The listing builds one solid part. Answer for the finished solid, in the listing's coordinates (mm). A direction names the side the tool comes from. Round coordinates to 2 decimals unless told otherwise and drop trailing zeros. Write each loop counter-clockwise with the first axis right and the second up, starting at its lowest first coordinate (ties: lowest second). Pieces come first, ordered by that corner, then holes. Notation, with made-up numbers: (64, -38) - (85, -38) arc R37 cw to (85, 1) - close; hole circle Ø5 at (19, -12.75). An arc over 180 degrees is marked (long way). Answer in a Markdown table with one row per item.
from build123d import *

# Parameters (mm, degrees)
SKETCH1_W           = 40
SKETCH1_H           = 35
SKETCH1_R           = 2.25
SKETCH1_W_2         = 6
SKETCH1_H_2         = 25
BOSS_EXTRUDE1_DEPTH = 4
SKETCH2_W           = 6
SKETCH2_H           = 25
BOSS_EXTRUDE2_DEPTH = 26
SKETCH3_R           = 2.35
CUT_EXTRUDE1_DEPTH  = 45.760529843
FILLET1_R           = 10
CHAMFER1_SIZE       = 1


with BuildPart() as part:
    # Sketch1 → Boss-Extrude1 (new body)
    with BuildSketch(Plane(origin=(0, 0, 0), x_dir=(1, 0, 0), z_dir=(0, 1, 0))):
        with Locations((-0.498134051, -0.87173459)):
            Rectangle(SKETCH1_W, SKETCH1_H)
        with Locations(Location((-12.118134051, -9.62173459, 0), (0, 0, 270))):
            Circle(SKETCH1_R, mode=Mode.SUBTRACT)
        with Locations(Location((-12.118134051, 7.87826541, 0), (0, 0, 270))):
            Circle(SKETCH1_R, mode=Mode.SUBTRACT)
        with Locations((10.881865949, -0.87173459)):
            Rectangle(SKETCH1_W_2, SKETCH1_H_2, mode=Mode.SUBTRACT)
    extrude(amount=BOSS_EXTRUDE1_DEPTH)

    # Sketch2 → Boss-Extrude2 (add)
    with BuildSketch(Plane(origin=(0, 4, 0), x_dir=(1, 0, 0), z_dir=(0, 1, 0))):
        with Locations((10.881865949, -0.87173459)):
            Rectangle(SKETCH2_W, SKETCH2_H)
    extrude(amount=-BOSS_EXTRUDE2_DEPTH)

    # Sketch3 → Cut-Extrude1 (cut, through all)
    with BuildSketch(Plane(origin=(13.881865949, 0, 0), x_dir=(0, 0, -1), z_dir=(1, 0, 0))):
        with Locations((6.12826541, -16.5)):
            Circle(SKETCH3_R)
        with Locations(Location((-7.87173459, -16.5, 0), (0, 0, 180))):
            Circle(SKETCH3_R)
    extrude(amount=-CUT_EXTRUDE1_DEPTH, mode=Mode.SUBTRACT)

    # Fillet1
    fillet1_edges = [part.edges().sort_by_distance(p)[0] for p in [
        (19.501865949, 2, 18.37173459),
        (-20.498134051, 2, 18.37173459),
        (-20.498134051, 2, -16.62826541),
        (19.501865949, 2, -16.62826541),
    ]]
    fillet(fillet1_edges, radius=FILLET1_R)

    # Chamfer1
    chamfer1_edges = [part.edges().sort_by_distance(p)[0] for p in [
        (-12.118134051, 0, 7.37173459),
        (-12.118134051, 4, 7.37173459),
        (-12.118134051, 0, -10.12826541),
        (-12.118134051, 4, -10.12826541),
        (7.881865949, -11, -11.62826541),
        (10.881865949, -22, -11.62826541),
        (13.881865949, -11, -11.62826541),
        (13.881865949, -22, 0.87173459),
        (13.881865949, -11, 13.37173459),
        (10.881865949, -22, 13.37173459),
        (7.881865949, -11, 13.37173459),
        (7.881865949, -22, 0.87173459),
        (7.881865949, -16.5, -3.77826541),
        (13.881865949, -16.5, -3.77826541),
        (7.881865949, -16.5, 5.52173459),
        (13.881865949, -16.5, 5.52173459),
        (19.501865949, 0, 0.87173459),
        (19.501865949, 4, 0.87173459),
        (-0.498134051, 0, 18.37173459),
        (-20.498134051, 0, 0.87173459),
        (-0.498134051, 0, -16.62826541),
        (-17.569201863, 0, 15.442802401),
        (-17.569201863, 0, -13.699333222),
        (16.572933761, 0, -13.699333222),
        (16.572933761, 0, 15.442802401),
        (-0.498134051, 4, 18.37173459),
        (-0.498134051, 4, -16.62826541),
        (-20.498134051, 4, 0.87173459),
        (-17.569201863, 4, 15.442802401),
        (-17.569201863, 4, -13.699333222),
        (16.572933761, 4, -13.699333222),
        (16.572933761, 4, 15.442802401),
    ]]
    chamfer(chamfer1_edges, length=CHAMFER1_SIZE)


solid = part.part
(1) Section B-B (z = -2) is taken. Give the vertices of the cut face in (x, y).
Checked values:
| item | result |
|---|---|
| outline | (-20.5, 1) - (-19.5, 0) - (7.88, 0) - (7.88, -21) - (8.88, -22) - (12.88, -22) - (13.88, -21) - (13.88, 0) - (18.5, 0) - (19.5, 1) - (19.5, 3) - (18.5, 4) - (-19.5, 4) - (-20.5, 3) - close |
(2) Section A-A (y = -16.5) is taken. Give the vertices of the cut face in (x, z).
Checked values:
| item | result |
|---|---|
| outline | (7.88, -10.63) - (8.88, -11.63) - (12.88, -11.63) - (13.88, -10.63) - (13.88, -9.48) - (12.88, -8.48) - (8.88, -8.48) - (7.88, -9.48) - close; (7.88, -2.78) - (8.88, -3.78) - (12.88, -3.78) - (13.88, -2.78) - (13.88, 4.52) - (12.88, 5.52) - (8.88, 5.52) - (7.88, 4.52) - close; (7.88, 11.22) - (8.88, 10.22) - (12.88, 10.22) - (13.88, 11.22) - (13.88, 12.37) - (12.88, 13.37) - (8.88, 13.37) - (7.88, 12.37) - close |
(3) For faces 4 (the flat face through (13.882, -10, 1)), 5 (the flat face through (13.389, -10.353, 12.865)), 6 (the flat face through (-0.36, 0.51, -16.14)), determine the directions among +Z, -Z, +X, -X, +Y, -Y from which every point of the face is accessible in a straight line to the end or side of a thin tool.
Checked values:
| item | result |
|---|---|
| face 4 | +Z, -Z, +X, -Y |
| face 5 | +Z, +X, -Y |
| face 6 | -Z, +X, -X, -Y |
(4) Section C-C (y = -3) is taken. Give the vertices of the cut face in (x, z).
Checked values:
| item | result |
|---|---|
| outline | (7.88, -10.63) - (8.88, -11.63) - (12.88, -11.63) - (13.88, -10.63) - (13.88, 12.37) - (12.88, 13.37) - (8.88, 13.37) - (7.88, 12.37) - close |
(5) Section D-D (x = -7) is taken. Give the vertices of the cut face in (y, z).
Checked values:
| item | result |
|---|---|
| outline | (0, -15.63) - (1, -16.63) - (3, -16.63) - (4, -15.63) - (4, 17.37) - (3, 18.37) - (1, 18.37) - (0, 17.37) - close |
(6) For a pull along Z with two mould halves and no side action, classify faces 1 (the cylindrical face through (10.91, -14.206, 7.362)), 2 (the flat face through (8.375, -10.353, -11.121)), 3 (the flat face through (-0.64, 0.51, 17.88)) as pulls with the +Z half, pulls with the -Z half, needs draft (parallel to the pull), parting line crosses it, or undercut.
Checked values:
| item | result |
|---|---|
| face 1 | undercut |
| face 2 | pulls with the -Z half |
| face 3 | pulls with the +Z half |
(7) Flat-ended cylindrical pins translate along their axes: pin 1 (1.5 mm diameter, centred on x = 9, y = -14.5, fed in from -Z); pin 2 (5.5 mm diameter, centred on y = -16.5, z = 7.87, fed in from -X); pin 3 (6.5 mm diameter, centred on y = -9.5, z = 5, fed in from +X). Find the tip coordinate at first contact, or state that the pin passes through.
Checked values:
| item | result |
|---|---|
| pin 1 | stops at z = -11.63 |
| pin 2 | stops at x = 8.48 |
| pin 3 | stops at x = 13.88 |
(8) Find the intervals of material crossed by line 1 (X direction, y = -8, z = -5.5); line 2 (Y direction, x = 18, z = -7.5); line 3 (X direction, y = 0.75, z = -8), in increasing order.
Checked values:
| item | result |
|---|---|
| line 1 | x = 7.88 to 13.88 |
| line 2 | y = 0 to 4 |
| line 3 | x = -20.15 to -14.62, -9.62 to 19.15 |
